```python
from build123d import *

# Parameters (mm, degrees)
SKETCH1_R           = 7.9375
BOSS_EXTRUDE1_DEPTH = 45.72
BOSS_EXTRUDE2_DEPTH = 6.35


with BuildPart() as part:
    # Sketch1 → Boss-Extrude1 (new body)
    with BuildSketch(Plane(origin=(0, 0, 0), x_dir=(1, 0, 0), z_dir=(0, 1, 0))):
        with Locations(Location((0, 0, 0), (0, 0, 270))):
            Circle(SKETCH1_R)
    extrude(amount=BOSS_EXTRUDE1_DEPTH)

    # Sketch2 → Boss-Extrude2 (add, symmetric)
    with BuildSketch(Plane(origin=(0, 44.341373311, -7.818580476), x_dir=(1, 0, 0), z_dir=(0, -0.9848077530122086, 0.17364817766692736))):
        with BuildLine():
            Line((-7.9375, 7.939194683), (7.9375, 7.939194683))
            Line((7.9375, 7.939194683), (12.7, 134.939194683))
            ThreePointArc((12.7, 134.939194683), (0, 147.639194683), (-12.7, 134.939194683))
            Line((-12.7, 134.939194683), (-7.9375, 7.939194683))
        make_face()
    extrude(amount=BOSS_EXTRUDE2_DEPTH, both=True)


solid = part.part
```
For this review, take the finished solid that the model builds, in its own axes (mm). A direction names the side the tool comes from. Coordinates: 2 decimals unless noted, no trailing zeros. Order: outer loops, then holes, each group sorted by start corner. A loop starts at its lowest first (then second) coordinate and runs counter-clockwise, first axis right, second up. Notation, with made-up numbers: (-38, 76) - (-25, 76) arc R12 ccw to (-25, 84) - close; hole circle Ø9 at (32.5, 32.25). An arc over 180 degrees is marked (long way). Answer as a JSON object with one key per item and string values. Group by question number.
1. We need section C-C on z = 26. State the section outline as (x, y) points, then the cut area to 3 significant figures.
2. We need section D-D on x = 6.5. State the section outline as (y, z) points.
3. For probe 1 along Z at (x, y) = (0.5, 34); probe 2 along Y at (x, z) = (6.5, 64.5); probe 3 along Z at (x, y) = (3.5, 32.5), list the stretches that pass through material, from the lowest coordinate up.
4. We need section B-B on y = 17. State the section outline as (x, z) points (1 decimal), then the cut area to 3 significant figures.
5. The part is to be moulded in two halves that separate along Y. For faces 3 (the cylindrical face through (0.28, 69.89, 137.59)), 4 (the flat face through (-0.111, 48.803, -0.544)), 5 (the flat face through (0, 0, 0)), 6 (the cylindrical face through (0.35, 22.54, -7.93)), say which applies: pulls with the +Y half, pulls with the -Y half, needs draft (parallel to the pull), parting line crosses it, or undercut.
6. Clearance check with flat-ended pins moving along their axes: P1, Ø4, axis at x = -1, z = 110.5, coming from the +Y side; P2, Ø5, axis at y = 47, z = 39, coming from the +X side; P3, Ø2.5, axis at x = -3, z = -4, coming from the +Y side; P4, Ø10, axis at x = 5, y = 28, coming from the -Z side. State where each tip first meets the part, or that it passes through.
7. For faces 1 (the flat face through (-0.178, 64.273, 68.649)), 2 (the flat face through (0, 45.72, -3)), list the 3-axis set-ups (+Z, -Z, +X, -X, +Y, -Y) from which the entire face can be reached by the end or side of a thin tool; tool diameter is ignored.
8. We need section A-A on x = 0. State the section outline as (y, z) points.
Final values:
{
 "1": {"outline": "(-8.97, 56.75) - (-8.89, 43.86) - (8.89, 43.86) - (8.97, 56.75) - close", "area": "230 mm²"},
 "2": {"outline": "(0, -4.56) - (45.72, -4.56) - (45.72, 0) - (51.97, -1.1) - (75.92, 134.71) - (63.41, 136.92) - (40.08, 4.56) - (0, 4.56) - close"},
 "3": {"probe 1": "-7.92 to 7.92", "probe 2": "50.65 to 63.54", "probe 3": "-7.12 to 7.12"},
 "4": {"outline": "circle Ø15.9 at (0, 0)", "area": "198 mm²"},
 "5": {"face 3": "pulls with the +Y half", "face 4": "undercut", "face 5": "pulls with the -Y half", "face 6": "needs draft"},
 "6": {"P1": "y = 72", "P2": "x = 9.48", "P3": "y = 45.72", "P4": "z = -7.94"},
 "7": {"face 1": "-Z, +X, -X, +Y", "face 2": "-Z, +X, -X"},
 "8": {"outline": "(0, -7.94) - (45.72, -7.94) - (45.72, 0) - (51.97, -1.1) - (76.23, 136.47) - (63.73, 138.68) - (40.67, 7.94) - (0, 7.94) - close"}
}
